from build123d import *

# Parameters (mm, degrees)
CROQUIS1_W              = 100
CROQUIS1_H              = 50
SALIENTE_EXTRUIR1_DEPTH = 10
CROQUIS2_W              = 87.380374462
CROQUIS2_H              = 39.837581604
SALIENTE_EXTRUIR2_DEPTH = 60
REDONDEO1_R             = 15
CROQUIS3_R              = 6.082397519
SALIENTE_EXTRUIR3_DEPTH = 10


with BuildPart() as part:
    # Croquis1 → Saliente-Extruir1 (new body)
    with BuildSketch(Plane(origin=(0, 0, 0), x_dir=(1, 0, 0), z_dir=(0, 1, 0))):
        Rectangle(CROQUIS1_W, CROQUIS1_H)
    extrude(amount=SALIENTE_EXTRUIR1_DEPTH)

    # Croquis2 → Saliente-Extruir2 (add)
    with BuildSketch(Plane(origin=(0, 10, 0), x_dir=(1, 0, 0), z_dir=(0, 1, 0))):
        Rectangle(CROQUIS2_W, CROQUIS2_H)
    extrude(amount=SALIENTE_EXTRUIR2_DEPTH)

    # Redondeo1
    redondeo1_edges = [part.edges().sort_by_distance(p)[0] for p in [
        (-43.690187231, 70, 0),
        (0, 70, 19.918790802),
        (43.690187231, 70, 0),
        (0, 70, -19.918790802),
    ]]
    fillet(redondeo1_edges, radius=REDONDEO1_R)

    # Croquis3 → Saliente-Extruir3 (add)
    with BuildSketch(Plane.XZ):
        with Locations(Location((0, 0, 0), (0, 0, 270))):
            Circle(CROQUIS3_R)
    extrude(amount=SALIENTE_EXTRUIR3_DEPTH)


solid = part.part
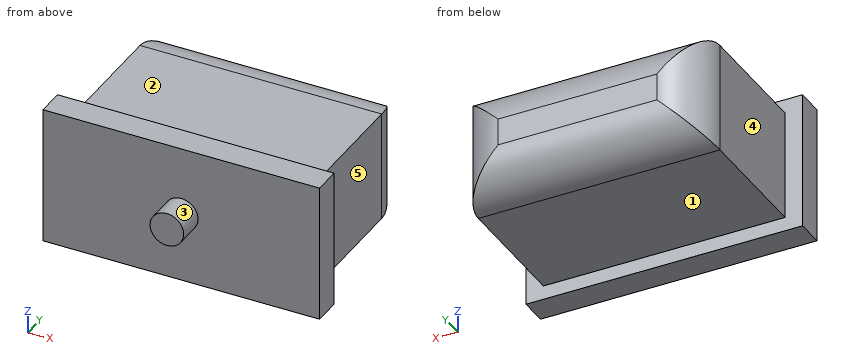
The model under review builds one solid part; all positions refer to its coordinate system, in mm. Face numbers are marked on the shaded views. A direction names the side the tool comes from. Give positions to 0.01 mm unless a question says otherwise; leave off trailing zeros. Write each loop counter-clockwise with the first axis right and the second up, starting at its lowest first coordinate (ties: lowest second). Pieces come first, ordered by that corner, then holes.
1. Add section A-A, the plane x = 0. Write out the cut boundary in (y, z).
2. Add section C-C, the plane y = 34. Write out the cut boundary in (x, z), plus the area to 3 significant figures.
3. Add section D-D, the plane x = -11.5. Write out the cut boundary in (y, z).
4. Add section B-B, the plane z = 0. Write out the cut boundary in (x, y).
5. For P1, Ø12, axis at y = 39, z = -6, coming from the +X side; P2, Ø4, axis at x = 31, y = 56, coming from the +Z side; P3, Ø6, axis at x = 38.5, z = -20, coming from the +Y side, all flat-tipped, find the tip position at first contact; note any pin that passes through.
6. Tool access review of the marked faces 1, 2, 3, 4 and 5: name each direction out of +Z, -Z, +X, -X, +Y, -Y from which nothing blocks a thin tool from reaching the whole face with its end or side.
7. Wall thickness on L1, parallel to Z at x = 36, y = 20; L2, parallel to Y at x = 23.5, z = 23; L3, parallel to X at y = 50.5, z = -19: over which ranges is each line inside the solid? List them lowest first.
Worked answers:
1. outline: (-10, -6.08) - (0, -6.08) - (0, -25) - (10, -25) - (10, -19.92) - (55, -19.92) arc R15 ccw to (70, -4.92) - (70, 4.92) arc R15 ccw to (55, 19.92) - (10, 19.92) - (10, 25) - (0, 25) - (0, 6.08) - (-10, 6.08) - close
2. outline: (-43.69, -19.92) - (43.69, -19.92) - (43.69, 19.92) - (-43.69, 19.92) - close
2. area: 3,480 mm2
3. outline: (0, -25) - (10, -25) - (10, -19.92) - (55, -19.92) arc R15 ccw to (70, -4.92) - (70, 4.92) arc R15 ccw to (55, 19.92) - (10, 19.92) - (10, 25) - (0, 25) - close
4. outline: (-50, 0) - (-6.08, 0) - (-6.08, -10) - (6.08, -10) - (6.08, 0) - (50, 0) - (50, 10) - (43.69, 10) - (43.69, 55) arc R15 ccw to (28.69, 70) - (-28.69, 70) arc R15 ccw to (-43.69, 55) - (-43.69, 10) - (-50, 10) - close
5. P1: stops at x = 43.69
5. P2: stops at z = 19.92
5. P3: stops at y = 63.89
6. face 1: -Z, +X, -X, +Y
6. face 2: +Z, +X, -X, +Y
6. face 3: -Y
6. face 4: +Z, -Z, -X, +Y
6. face 5: +Z, -Z, +X, +Y
7. L1: z = -19.92 to 19.92
7. L2: y = 0 to 10
7. L3: x = -43.69 to 43.69
